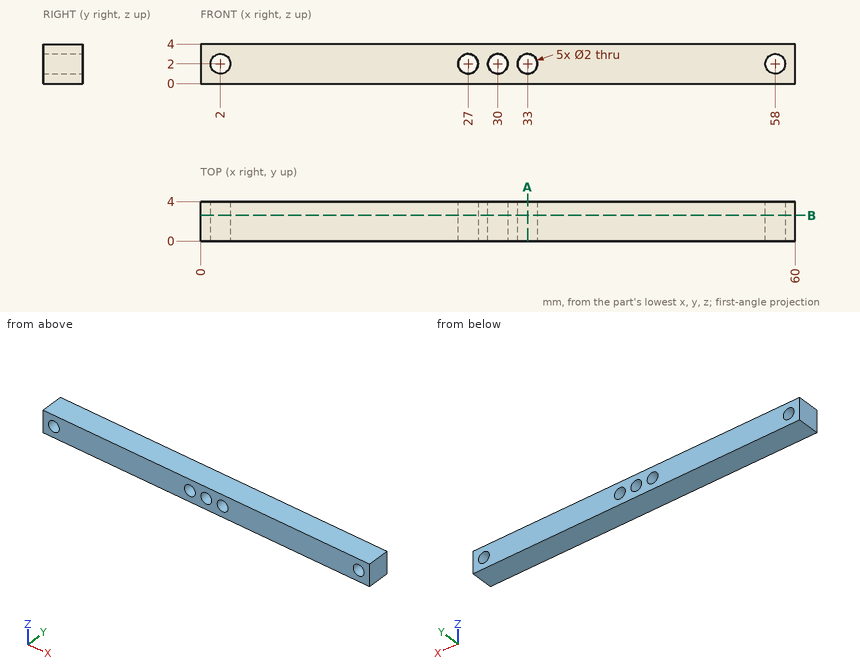
Drawing for the job (mm, zero at the part's lowest x, y, z). Round coordinates to 2 decimals unless told otherwise and drop trailing zeros. Write each loop counter-clockwise with the first axis right and the second up, starting at its lowest first coordinate (ties: lowest second). Pieces come first, ordered by that corner, then holes. Notation, with made-up numbers: (-7, 27.5) - (19, 27.5) arc R26 ccw to (19, 47.5) - close; hole circle Ø9 at (32, -9.5). An arc over 180 degrees is marked (long way). Return JSON: item names as keys, results as strings. Group by question number.
Item 1: Flat gauge pin, fed straight in: pin 1 Ø1.2 at (x, z) = (2, 2) entering from +Y. Where does the tip first touch, or does it go through?
Item 2: Band-saw the part on A-A on x = 33. List the corners of the cut face in (y, z), plus the area to 3 significant figures.
Item 3: Band-saw the part on B-B on y = 2.6. List the corners of the cut face in (x, z), plus the area to 3 significant figures.
Item 4: Probe probe 1 along X at (y, z) = (3.25, 2); probe 2 along X at (y, z) = (3.75, 2.4); probe 3 along Z at (x, y) = (58, 2.4). List the from-to ranges inside material, lowest first.
Resolved:
{
 "1": {"pin 1": "passes through"},
 "2": {"outline": "(0, 0) - (4, 0) - (4, 1) - (0, 1) - close; (0, 3) - (4, 3) - (4, 4) - (0, 4) - close", "area": "8.00 mm²"},
 "3": {"outline": "(0, 0) - (60, 0) - (60, 4) - (0, 4) - close; hole circle Ø2 at (2, 2); hole circle Ø2 at (27, 2); hole circle Ø2 at (30, 2); hole circle Ø2 at (33, 2); hole circle Ø2 at (58, 2)", "area": "224 mm²"},
 "4": {"probe 1": "x = 0 to 1, 3 to 26, 28 to 29, 31 to 32, 34 to 57, 59 to 60", "probe 2": "x = 0 to 1.08, 2.92 to 26.08, 27.92 to 29.08, 30.92 to 32.08, 33.92 to 57.08, 58.92 to 60", "probe 3": "z = 0 to 1, 3 to 4"}
}
